from build123d import *

# Parameters (mm, degrees)
SKETCH1_W           = 508
SKETCH1_H           = 25.4
BOSS_EXTRUDE1_DEPTH = 12.7
SKETCH2_R           = 9.525
CUT_EXTRUDE1_DEPTH  = 255.634208228
SKETCH3_R           = 9.525
BOSS_EXTRUDE2_DEPTH = 76.2


with BuildPart() as part:
    # Sketch1 → Boss-Extrude1 (new body)
    with BuildSketch(Plane(origin=(0, 0, 0), x_dir=(1, 0, 0), z_dir=(0, 1, 0))):
        Rectangle(SKETCH1_W, SKETCH1_H)
    extrude(amount=BOSS_EXTRUDE1_DEPTH)

    # Sketch2 → Cut-Extrude1 (cut, through all)
    with BuildSketch(Plane(origin=(0, 12.7, 0), x_dir=(1, 0, 0), z_dir=(0, 1, 0))):
        with Locations(Location((-228.6, 0, 0), (0, 0, 270))):
            Circle(SKETCH2_R)
        with Locations(Location((228.6, 0, 0), (0, 0, 90))):
            Circle(SKETCH2_R)
    extrude(amount=-CUT_EXTRUDE1_DEPTH, mode=Mode.SUBTRACT)

    # Sketch3 → Boss-Extrude2 (add)
    with BuildSketch(Plane.XZ):
        with Locations(Location((-127, 0, 0), (0, 0, 90))):
            Circle(SKETCH3_R)
        with Locations(Location((127, 0, 0), (0, 0, 90))):
            Circle(SKETCH3_R)
    extrude(amount=BOSS_EXTRUDE2_DEPTH)


solid = part.part
Can you work these out from the model? Positions are in its coordinate system, mm. Coordinates: 2 decimals unless noted, no trailing zeros. Write each loop counter-clockwise with the first axis right and the second up, starting at its lowest first coordinate (ties: lowest second). Pieces come first, ordered by that corner, then holes. Notation, with made-up numbers: (33.25, 31) -> (70.25, 31) arc R17 ccw to (70.25, 60) -> close; hole circle Ø7 at (59, 62.25). An arc over 180 degrees is marked (long way). Write each question's results on one line, items separated by ' | '. Start each with the question number.
Item 1: Thinking about a two-plate mould opening in X: for faces 1 (the cylindrical face through (117.556, -37.567, -1.24)), 2 (the cylindrical face through (-136.444, -37.567, -1.24)), 3 (the flat face through (254, 6, 0)), 4 (the flat face through (-254, 6, 0)), which applies, released by +X, released by -X, zero draft, split by the parting line, or undercut?
Item 2: If we section it at C-C, the plane x = 127: Write out the boundary of the cut face in (y, z) (3 decimals), and give its area (3 significant figures).
Item 3: If we section it at D-D, the plane y = -37: Write out the boundary of the cut face in (x, z) (3 decimals).
Item 4: If we section it at B-B, the plane x = 228.6: Write out the boundary of the cut face in (y, z) (3 decimals), and give its area (3 significant figures).
Item 5: If we section it at A-A, the plane z = -1.5: Write out the boundary of the cut face in (x, y), and give its area (3 significant figures).
Item 6: I'm going to push flat-ended pins straight in: P1, Ø12, axis at x = 118, y = -26, coming from the +Z side; P2, Ø8, axis at y = -65, z = -7.5, coming from the +X side; P3, Ø10, axis at y = -65, z = -8, coming from the +X side. Where does each tip first touch, or does it pass through?
Item 7: Please list where these lines run through material, in increasing order: probe 1 along X at (y, z) = (8.25, 0) (3 decimals); probe 2 along X at (y, z) = (7, 1.25); probe 3 along Z at (x, y) = (228, 7).
Answer block:
1) face 1: undercut | face 2: undercut | face 3: released by +X | face 4: released by -X
2) outline: (-76.2, -9.525) -> (0, -9.525) -> (0, -12.7) -> (12.7, -12.7) -> (12.7, 12.7) -> (0, 12.7) -> (0, 9.525) -> (-76.2, 9.525) -> close | area: 1,770 mm²
3) outline: circle Ø19.05 at (-127, 0); circle Ø19.05 at (127, 0)
4) outline: (0, -12.7) -> (12.7, -12.7) -> (12.7, -9.525) -> (0, -9.525) -> close; (0, 9.525) -> (12.7, 9.525) -> (12.7, 12.7) -> (0, 12.7) -> close | area: 80.6 mm²
5) outline: (-254, 0) -> (-238.01, 0) -> (-238.01, 12.7) -> (-254, 12.7) -> close; (-219.19, 0) -> (-136.41, 0) -> (-136.41, -76.2) -> (-117.59, -76.2) -> (-117.59, 0) -> (117.59, 0) -> (117.59, -76.2) -> (136.41, -76.2) -> (136.41, 0) -> (219.19, 0) -> (219.19, 12.7) -> (-219.19, 12.7) -> close; (238.01, 0) -> (254, 0) -> (254, 12.7) -> (238.01, 12.7) -> close | area: 8,840 mm²
6) P1: z = 9.04 | P2: x = 135.86 | P3: x = 136.04
7) probe 1: -254 to -238.125, -219.075 to 219.075, 238.125 to 254 | probe 2: -254 to -238.04, -219.16 to 219.16, 238.04 to 254 | probe 3: -12.7 to -9.51, 9.51 to 12.7
